Read the model definition and answer for the solid it produces. Units are mm, in the model's axes. Coordinates: 2 decimals unless noted, no trailing zeros. Loops run counter-clockwise (first coordinate to the right, second up) from the corner with the lowest first, then second, coordinate; pieces in that order, holes last. Notation, with made-up numbers: M -4.5,59.5 L 13.5,59.5 A25 ccw 13.5,86.5 Z; hole C 13,62.25 d1. An arc over 180 degrees is marked long. Put each result on its own line as item: value.
from build123d import *

# Parameters (mm, degrees)
BOSS_EXTRUDE1_DEPTH      = 7
SKETCH2_R                = 5
CUT_EXTRUDE1_DEPTH       = 7
LPATTERN1_COUNT          = 7
LPATTERN1_PITCH          = 30
SKETCH6_R                = 5
CUT_EXTRUDE2_DEPTH       = 10
CUT_EXTRUDE4_REACH       = 219.196
SKETCH9_R                = 1.5
SKETCH16_W               = 47
SKETCH16_H               = 39.930416712
SKETCH16_R               = 8.2
BOSS_EXTRUDE2_DEPTH      = 10
SKETCH17_W               = 45.833760325
SKETCH17_H               = 30.12512517
SKETCH17_W_2             = 13.763297709
SKETCH17_H_2             = 9.222578979
CUT_EXTRUDE15_DEPTH      = 9
CUT_EXTRUDE18_REACH      = 223.779
SKETCH18_W               = 140
SKETCH18_H               = 115.832892108
BOSS_EXTRUDE5_START      = -7
BOSS_EXTRUDE5_DEPTH      = 7
CUT_EXTRUDE19_DEPTH      = 10
SKETCH25_W               = 7
SKETCH25_H               = 3
BOSS_EXTRUDE6_DEPTH      = 12.7
CUT_EXTRUDE20_DEPTH      = 114.382079461
CUT_EXTRUDE20_DEPTH_BACK = 114.382079461
SKETCH26_R               = 1.5


with BuildPart() as part:
    # Sketch1 → Boss-Extrude1 (new body)
    with BuildSketch(Plane.XY):
        with BuildLine():
            Line((-200, 0), (50, 0))
            ThreePointArc((50, 0), (65, -15), (50, -30))
            Line((50, -30), (-200, -30))
            ThreePointArc((-200, -30), (-215, -15), (-200, 0))
        make_face()
    extrude(amount=BOSS_EXTRUDE1_DEPTH)

    # Sketch2 → Cut-Extrude1 (cut)
    with BuildSketch(Plane.XY.offset(7)):
        with Locations((-185, -15)):
            Circle(SKETCH2_R)
    cut_extrude1 = extrude(amount=-CUT_EXTRUDE1_DEPTH, mode=Mode.SUBTRACT)

    # LPattern1: Cut-Extrude1 ×7
    with Locations(*[(i * LPATTERN1_PITCH, 0, 0) for i in range(1, LPATTERN1_COUNT)]):
        add(cut_extrude1, mode=Mode.SUBTRACT)

    # Sketch6 → Cut-Extrude2 (cut)
    with BuildSketch(Plane(origin=(0, 0, 0), x_dir=(-1, 0, 0), z_dir=(0, 0, -1))):
        with Locations((-50, -15)):
            Circle(SKETCH6_R)
    extrude(amount=-CUT_EXTRUDE2_DEPTH, mode=Mode.SUBTRACT)

    # Sketch9 → Cut-Extrude4 (cut, up to next)
    with BuildSketch(Plane(origin=(0, 0, 0), x_dir=(-1, 0, 0), z_dir=(0, 0, -1)), mode=Mode.PRIVATE) as cut_extrude4_sk1:
        with Locations((-29.5, -6.25)):
            Circle(SKETCH9_R)
    cut_extrude4_tool1 = extrude(cut_extrude4_sk1.sketch, amount=-CUT_EXTRUDE4_REACH, mode=Mode.PRIVATE) & part.part
    # Sketch9 → Cut-Extrude4 (cut, up to next)
    with BuildSketch(Plane(origin=(0, 0, 0), x_dir=(-1, 0, 0), z_dir=(0, 0, -1)), mode=Mode.PRIVATE) as cut_extrude4_sk2:
        with Locations((-29.5, -23.75)):
            Circle(SKETCH9_R)
    cut_extrude4_tool2 = extrude(cut_extrude4_sk2.sketch, amount=-CUT_EXTRUDE4_REACH, mode=Mode.PRIVATE) & part.part
    add(cut_extrude4_tool1.solids().sort_by_distance((29.5, -6.25, 0))[0], mode=Mode.SUBTRACT)
    add(cut_extrude4_tool2.solids().sort_by_distance((29.5, -23.75, 0))[0], mode=Mode.SUBTRACT)

    # Sketch16 → Boss-Extrude2 (add)
    with BuildSketch(Plane(origin=(0, 0, 0), x_dir=(-1, 0, 0), z_dir=(0, 0, -1))):
        with Locations((156.5, -31.726084321)):
            Rectangle(SKETCH16_W, SKETCH16_H)
        with Locations((143.645834005, -39.243444981)):
            Circle(SKETCH16_R, mode=Mode.SUBTRACT)
        with Locations((169.806394215, -39.243444981)):
            Circle(SKETCH16_R, mode=Mode.SUBTRACT)
        with BuildLine():
            Line((152.543612389, -45.175236858), (161.148055619, -45.175236858))
            ThreePointArc((161.148055619, -45.175236858), (162.890378664, -46.917559902), (161.148055619, -48.659882947))
            Line((161.148055619, -48.659882947), (152.543612389, -48.659882947))
            ThreePointArc((152.543612389, -48.659882947), (150.801289344, -46.917559902), (152.543612389, -45.175236858))
        make_face(mode=Mode.SUBTRACT)
    extrude(amount=BOSS_EXTRUDE2_DEPTH)

    # Sketch17 → Cut-Extrude15 (cut)
    with BuildSketch(Plane(origin=(0, 0, -10), x_dir=(-1, 0, 0), z_dir=(0, 0, -1))):
        with Locations((156.666880163, -35.963336462)):
            Rectangle(SKETCH17_W, SKETCH17_H)
        with Locations((156.826506841, -16.372165454)):
            Rectangle(SKETCH17_W_2, SKETCH17_H_2)
    extrude(amount=-CUT_EXTRUDE15_DEPTH, mode=Mode.SUBTRACT)

    # Sketch18 → Cut-Extrude18 (cut, up to next)
    with BuildSketch(Plane.XY.offset(7), mode=Mode.PRIVATE) as cut_extrude18_sk1:
        with Locations((-145, -15)):
            Rectangle(SKETCH18_W, SKETCH18_H)
    cut_extrude18_tool1 = extrude(cut_extrude18_sk1.sketch, amount=-CUT_EXTRUDE18_REACH, mode=Mode.PRIVATE) & part.part
    add(cut_extrude18_tool1.solids().sort_by_distance((-145, -15, 7))[0], mode=Mode.SUBTRACT)

    # Sketch23 → Boss-Extrude5 (add)
    with BuildSketch(Plane.XY.offset(7).offset(BOSS_EXTRUDE5_START)):
        with BuildLine():
            Line((95, 0), (50, 0))
            ThreePointArc((50, 0), (65, -15), (50, -30))
            Line((50, -30), (95, -30))
            ThreePointArc((95, -30), (110, -15), (95, 0))
        make_face()
    extrude(amount=BOSS_EXTRUDE5_DEPTH)

    # Sketch24 → Cut-Extrude19 (cut)
    with BuildSketch(Plane.XY.offset(7)):
        with BuildLine():
            ThreePointArc((87.45, -25), (87.010660172, -23.939339828), (85.95, -23.5))
            Line((85.95, -23.5), (85.95, -26.5))
            ThreePointArc((85.95, -26.5), (87.010660172, -26.060660172), (87.45, -25))
        make_face()
        with BuildLine():
            Line((85.95, -26.5), (85.95, -23.5))
            ThreePointArc((85.95, -23.5), (84.45, -25), (85.95, -26.5))
        make_face()
        with BuildLine():
            ThreePointArc((87.45, -5), (87.010660172, -3.939339828), (85.95, -3.5))
            Line((85.95, -3.5), (85.95, -6.5))
            ThreePointArc((85.95, -6.5), (87.010660172, -6.060660172), (87.45, -5))
        make_face()
        with BuildLine():
            Line((85.95, -6.5), (85.95, -3.5))
            ThreePointArc((85.95, -3.5), (84.45, -5), (85.95, -6.5))
        make_face()
    extrude(amount=-CUT_EXTRUDE19_DEPTH, mode=Mode.SUBTRACT)

    # Sketch25 → Boss-Extrude6 (add)
    with BuildSketch(Plane.ZY.offset(75)):
        with Locations((3.5, -4.920008597)):
            Rectangle(SKETCH25_W, SKETCH25_H)
        with Locations((3.5, -24.2)):
            Rectangle(SKETCH25_W, SKETCH25_H)
    extrude(amount=BOSS_EXTRUDE6_DEPTH)

    # Sketch26 → Cut-Extrude20 (cut, two sides: drawn at the far end of the back side and taken through both)
    with BuildSketch(Plane(origin=(0, -3.420008597, 0), x_dir=(1, 0, 0), z_dir=(0, 1, 0)).offset(-CUT_EXTRUDE20_DEPTH_BACK)):
        with Locations(Location((-81.1, -3.5, 0), (0, 0, 180))):
            Circle(SKETCH26_R)
    extrude(amount=CUT_EXTRUDE20_DEPTH + CUT_EXTRUDE20_DEPTH_BACK, mode=Mode.SUBTRACT)


solid = part.part
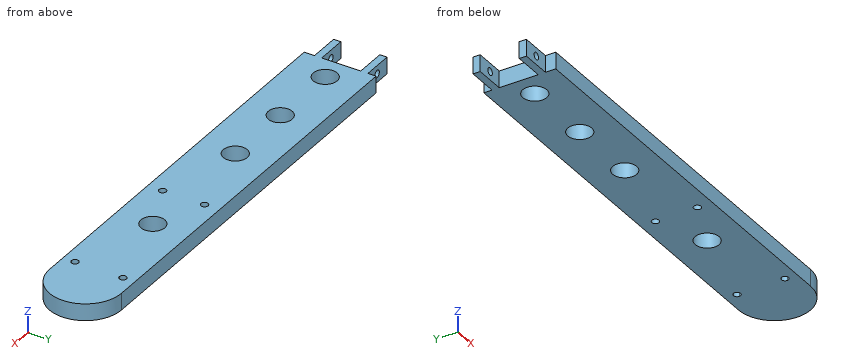
1) Straight lines are drawn through the part: line 1 (Y direction, x = 29.5, z = 2); line 2 (X direction, y = -17.75, z = 5.25); line 3 (X direction, y = -24.25, z = 3.5). For each, find the intervals that lie inside material, in ascending order. Write a range as [from, to].
Answer list:
line 1: y = [-30, -25.25], [-22.25, -7.75], [-4.75, 0]
line 2: x = [-75, -69.18], [-60.82, -39.18], [-30.82, -9.18], [-0.82, 45.82], [54.18, 109.75]
line 3: x = [-87.7, -82.6], [-79.6, 28.09], [30.91, 84.65], [87.25, 106.81]
2) Find section A-A, the plane y = -15. Write down the section's boundary in (x, z).
Answer list:
outline: M -75,0 L -70,0 L -70,7 L -75,7 Z; M -60,0 L -40,0 L -40,7 L -60,7 Z; M -30,0 L -10,0 L -10,7 L -30,7 Z; M 0,0 L 45,0 L 45,7 L 0,7 Z; M 55,0 L 110,0 L 110,7 L 55,7 Z
3) Given pin 1 Ø1.3 at (y, z) = (-27, 4.5) entering from -X; pin 2 Ø3.5 at (x, z) = (-80, 2) entering from -Y, each flat-ended and moving along its own axis, determine where each tip first touches the part or whether it passes through.
Answer list:
pin 1: stops at x = -75
pin 2: stops at y = -25.7
4) Find section B-B, the plane x = -5. Write down the section's boundary in (y, z).
Answer list:
outline: M -30,0 L -20,0 L -20,7 L -30,7 Z; M -10,0 L 0,0 L 0,7 L -10,7 Z
